Read the model definition and answer for the solid it produces. Units are mm, in the model's axes. A direction names the side the tool comes from. Give positions to 0.01 mm unless a question says otherwise; leave off trailing zeros. Order: outer loops, then holes, each group sorted by start corner. A loop starts at its lowest first (then second) coordinate and runs counter-clockwise, first axis right, second up. Notation, with made-up numbers: (52.5, 22) - (85.5, 22) arc R6 ccw to (85.5, 31) - close; hole circle Ø1 at (19.25, 73). An arc over 180 degrees is marked (long way). Return JSON: item names as keys, results as strings.
```python
from build123d import *

# Parameters (mm, degrees)
SCHIZZO4_W  = 25
SCHIZZO4_H  = 30
SCHIZZO5_W  = 7
SCHIZZO5_H  = 40.640509339
RACCORDO1_R = 10


with BuildPart() as part:
    # Schizzo1 → Rivoluzione1 (revolve)
    with BuildSketch(Plane.XY, mode=Mode.PRIVATE) as rivoluzione1_sk:
        Polygon((-32.234492396, 0), (-12.5, 73.650128282), (-12.5, 81.650128282), (-25.490381057, 94.640509339), (-63, 94.640509339), (-38, 64.640509339), (-38, 0), align=None)
    revolve(rivoluzione1_sk.sketch.rotate(Axis((0, 0, 0), (0, 1, 0)), 270), axis=Axis((0, 0, 0), (0, 1, 0)))

    # Schizzo4 → Taglia-Rivoluzione3 (revolve, cut)
    with BuildSketch(Plane.XY, mode=Mode.PRIVATE) as taglia_rivoluzione3_sk:
        with Locations((-50.5, 79.640509339)):
            Rectangle(SCHIZZO4_W, SCHIZZO4_H)
    revolve(taglia_rivoluzione3_sk.sketch.rotate(Axis((0, 0, 0), (0, 1, 0)), 270), axis=Axis((0, 0, 0), (0, 1, 0)), mode=Mode.SUBTRACT)

    # Schizzo5 → Rivoluzione2 (revolve)
    with BuildSketch(Plane.XY, mode=Mode.PRIVATE) as rivoluzione2_sk:
        with Locations((-41.5, 74.32025467)):
            Rectangle(SCHIZZO5_W, SCHIZZO5_H)
        Polygon((-38, 54), (-38, 47), (-45, 54), align=None)
    revolve(rivoluzione2_sk.sketch.rotate(Axis((0, 0, 0), (0, 1, 0)), 270), axis=Axis((0, 0, 0), (0, 1, 0)))

    # Raccordo1
    raccordo1_edges = [part.edges().sort_by_distance(p)[0] for p in [
        (0, 47, 38),
    ]]
    fillet(raccordo1_edges, radius=RACCORDO1_R)


solid = part.part
```
Q1. Determine the mould class of faces 1 (the flat face through (19, 94.641, -19)), 2 (the cylindrical face through (17.235, 74.605, -41.569)), 3 (the conical face through (12.996, 82.463, 2.886)) for opening direction X: released by +X, released by -X, zero draft, split by the parting line, or undercut.
Values:
{"face 1": "zero draft", "face 2": "split by the parting line", "face 3": "undercut"}
Q2. Given pin 1 (12 mm diameter, centred on y = 24.5, z = -8.5, fed in from -X); pin 2 (5 mm diameter, centred on x = -24, y = 11.5, fed in from +Z); pin 3 (22.5 mm diameter, centred on x = 0, z = 0, fed in from +Y); pin 4 (8 mm diameter, centred on x = -16.5, y = 68, fed in from +Z), each flat-ended and moving along its own axis, determine where each tip first touches the part or whether it passes through.
Values:
{"pin 1": "stops at x = -37.92", "pin 2": "stops at z = 31.33", "pin 3": "passes through", "pin 4": "stops at z = 43.23"}
Q3. A cutting plane is placed at B-B (y = 12). Write down the section's boundary in (x, z), and give its area (3 significant figures).
Values:
{"outline": "circle Ø76 at (0, 0); hole circle Ø58.04 at (0, 0)", "area": "1,890 mm²"}
Q4. A cutting plane is placed at A-A (y = 33). Write down the section's boundary in (x, z), and give its area (3 significant figures).
Values:
{"outline": "circle Ø76 at (0, 0); hole circle Ø46.78 at (0, 0)", "area": "2,820 mm²"}
Q5. Consider L1, parallel to X at y = 77.75, z = 0; L2, parallel to Z at x = 5.5, y = 62.5; L3, parallel to Z at x = -5, y = 84. Determine where each line is inside the solid, lowest interval first.
Values:
{"L1": "x = -45 to -12.5, 12.5 to 45", "L2": "z = -44.66 to -14.48, 14.48 to 44.66", "L3": "z = -44.72 to -13.98, 13.98 to 44.72"}
Q6. For faces 4 (the cylindrical face through (-3.755, 77.706, -11.923)), 5 (the cylindrical face through (23.122, 21.129, 30.156)), determine the directions among +Z, -Z, +X, -X, +Y, -Y from which every point of the face is accessible in a straight line to the end or side of a thin tool.
Values:
{"face 4": "+Y, -Y", "face 5": "-Y"}
